Design review of the part built by this model. Coordinates are the model's own, in mm. Face numbers are marked on the shaded views. A direction names the side the tool comes from. Round coordinates to 2 decimals unless told otherwise and drop trailing zeros. Order: outer loops, then holes, each group sorted by start corner. A loop starts at its lowest first (then second) coordinate and runs counter-clockwise, first axis right, second up. Notation, with made-up numbers: (44, -23) - (81, -23) arc R23 ccw to (81, -11) - close; hole circle Ø8 at (41, 52.25). An arc over 180 degrees is marked (long way). Write item = value, one per line.
from build123d import *

# Parameters (mm, degrees)
SKETCH_1_W           = 150
SKETCH_1_H           = 25
EXTRUDE_1_DEPTH      = 70
SKETCH_2_R           = 7
CUT_EXTRUDE_1_DEPTH  = 168.406690428
EXTRUDE_START        = -80
SKETCH_3_R           = 17.5
EXTRUDE_2_DEPTH      = 15
EXTRUDE_5_DEPTH      = 5
EXTRUDE_5_DEPTH_BACK = 5


with BuildPart() as part:
    # Эскиз1 → Бобышка-Вытянуть1 (new body)
    with BuildSketch(Plane.XY):
        with Locations((75, -12.5)):
            Rectangle(SKETCH_1_W, SKETCH_1_H)
    extrude(amount=EXTRUDE_1_DEPTH)

    # Эскиз2 → Вырез-Вытянуть1 (cut, through all)
    with BuildSketch(Plane(origin=(0, 0, 0), x_dir=(1, 0, 0), z_dir=(0, 1, 0))):
        with BuildLine():
            Line((18, -24), (0, -24))
            Line((0, -24), (0, -46))
            Line((0, -46), (18, -46))
            ThreePointArc((18, -46), (29, -35), (18, -24))
        make_face()
        with Locations(Location((130, -12, 0), (0, 0, 270))):
            Circle(SKETCH_2_R)
        with Locations(Location((130, -58, 0), (0, 0, 270))):
            Circle(SKETCH_2_R)
    extrude(amount=-CUT_EXTRUDE_1_DEPTH, mode=Mode.SUBTRACT)

    # Эскиз3 → Бобышка-Вытянуть2 (add)
    with BuildSketch(Plane(origin=(150, 0, 0), x_dir=(0, 0, -1), z_dir=(1, 0, 0)).offset(EXTRUDE_START)):
        with BuildLine():
            Line((-70, 0), (-70, 47))
            ThreePointArc((-70, 47), (-35, 82), (0, 47))
            Line((0, 47), (0, 0))
            Line((0, 0), (-70, 0))
        make_face()
        with Locations((-35, 47)):
            Circle(SKETCH_3_R, mode=Mode.SUBTRACT)
    extrude(amount=-EXTRUDE_2_DEPTH)

    # Sketch 1 2 → Бобышка-Вытянуть5 (add, two sides: drawn at the far end of the back side and taken through both)
    with BuildSketch(Plane(origin=(70, 27, 35), x_dir=(0.8288486740756482, -0.5594728550010625, 0), z_dir=(0, 0, -1)).offset(-EXTRUDE_5_DEPTH_BACK)):
        Polygon((0, 0), (48.259714048, 0), (15.105767085, 22.3789142), align=None)
    extrude(amount=EXTRUDE_5_DEPTH + EXTRUDE_5_DEPTH_BACK)


solid = part.part
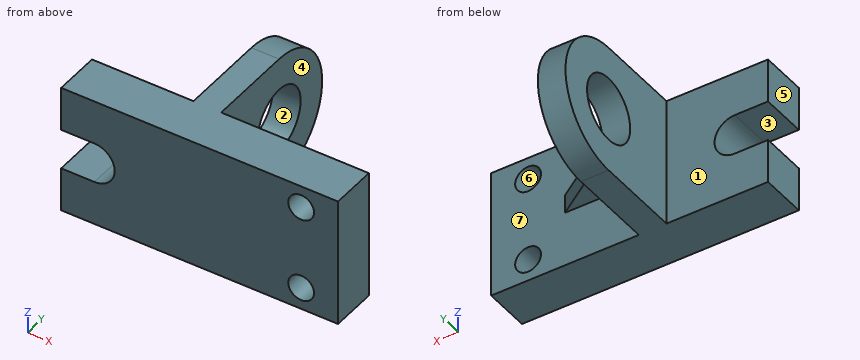
Item 1: The part is to be moulded in two halves that separate along X. For the marked faces 5, 6 and 7, say which applies: +X half, -X half, draft (parallel to the pull), parting line (faces both ways), or undercut.
Data:
face_5 = -X half
face_6 = undercut
face_7 = draft
Item 2: Take a section at C-C, the plane y = -10. State the section outline as (x, z) points.
Data:
outline = (0, 0) - (150, 0) - (150, 70) - (0, 70) - (0, 46) - (18, 46) arc R11 cw to (18, 24) - (0, 24) - close; hole circle Ø14 at (130, 12); hole circle Ø14 at (130, 58)
Item 3: Take a section at A-A, the plane z = 35. State the section outline as (x, y) points.
Data:
outline = (29, -25) - (150, -25) - (150, 0) - (110, 0) - (70, 27) - (70, 29.5) - (55, 29.5) - (55, 0) - (29, 0) - close; (55, 64.5) - (70, 64.5) - (70, 82) - (55, 82) - close
Item 4: Take a section at B-B, the plane x = 130. State the section outline as (y, z) points, and give its area (3 significant figures).
Data:
outline = (-25, 0) - (0, 0) - (0, 5) - (-25, 5) - close; (-25, 19) - (0, 19) - (0, 51) - (-25, 51) - close; (-25, 65) - (0, 65) - (0, 70) - (-25, 70) - close
area = 1,050 mm2
Item 5: For line 1 along X through (y, z) = (-8, 58); line 2 along Y through (x, z) = (101.5, 26.5); line 3 along X through (y, z) = (52, 13.5), list the stretches that pass through material, from the lowest coordinate up. Write a range as [from, to].
Data:
line_1 = [0, 123], [137, 150]
line_2 = [-25, 0]
line_3 = [55, 70]
Item 6: Insertion check: P1, Ø21.5, axis at x = 92.5, y = 13.5, coming from the -Z side; P2, Ø13.5, axis at x = 81.5, y = 15.5, coming from the +Z side; P3, Ø10, axis at y = 14, z = 48.5, coming from the +X side; P4, Ø11, axis at x = 130, z = 58, coming from the +Y side. Each pin has a flat end and moves straight along its axis. Give the tip position at first contact, or say it passes through.
Data:
P1 = 30
P2 = 40
P3 = 70
P4 = through
Item 7: For the marked faces 1, 2, 3 and 4, list the 3-axis set-ups (+Z, -Z, +X, -X, +Y, -Y) from which the entire face can be reached by the end or side of a thin tool; tool diameter is ignored.
Data:
face_1 = +Z, -Z, -X, +Y
face_2 = +X, -X
face_3 = -X, +Y, -Y
face_4 = +X, +Y
Item 8: Take a section at D-D, the plane y = 51. State the section outline as (x, z) points, and give its area (3 significant figures).
Data:
outline = (55, 0.23) - (70, 0.23) - (70, 17.96) - (55, 17.96) - close; (55, 52.04) - (70, 52.04) - (70, 69.77) - (55, 69.77) - close
area = 532 mm2
